Design review of the part built by this model. Coordinates are the model's own, in mm. Face numbers are marked on the shaded views. Round coordinates to 2 decimals unless told otherwise and drop trailing zeros. Loops run counter-clockwise (first coordinate to the right, second up) from the corner with the lowest first, then second, coordinate; pieces in that order, holes last. Notation, with made-up numbers: (46.5, -15) - (84.5, -15) arc R16 ccw to (84.5, 11) - close; hole circle Ø6 at (82.5, 85.5). An arc over 180 degrees is marked (long way). Return JSON: item names as keys, results as strings. Group by question number.
Autodesk Inventor part; units mm, degrees
ref_plane "YZ Plane" through (0, 0, 0) normal (1, 0, 0) x (0, 1, 0)
ref_plane "XZ Plane" through (0, 0, 0) normal (0, 1, 0) x (-1, 0, 0)
ref_plane "XY Plane" through (0, 0, 0) normal (0, 0, 1) x (1, 0, 0)
sketch "スケッチ1" plane through (0, 0, 0) normal (0, 0, 1) x (1, 0, 0)
  circle A0 centre (0, 0) radius 1.5
  dimension "d0" = 3
extrude "押し出し1" add sketch "スケッチ1" along normal blind 12
thread "ねじ1"
sketch "スケッチ2" plane through (0, 0, 12) normal (0, 0, 1) x (1, 0, 0)
  circle A0 centre (0, 0) radius 3
  dimension "d5" = 6
extrude "押し出し2" add sketch "スケッチ2" against normal blind 1.75
chamfer "面取り1" distance 1.5 angle 45 1 edges at (-3, 0, 10.25)
sketch "スケッチ3" plane through (0, 0, 12) normal (0, 0, 1) x (1, 0, 0)
  line L0 (0, 1.1547) -> (1, 0.5774)
  line L1 (1, 0.5774) -> (1, -0.5774)
  line L2 (1, -0.5774) -> (0, -1.1547)
  line L3 (0, -1.1547) -> (-1, -0.5774)
  line L4 (-1, -0.5774) -> (-1, 0.5774)
  line L5 (-1, 0.5774) -> (0, 1.1547)
  point P0 (0, 0)
  point P1 (0, 0)
  dimension "d11" = 2
extrude "押し出し3" cut sketch "スケッチ3" against normal blind 1.5
properties part number "m3皿ネジ12" material "鉄 灰色"
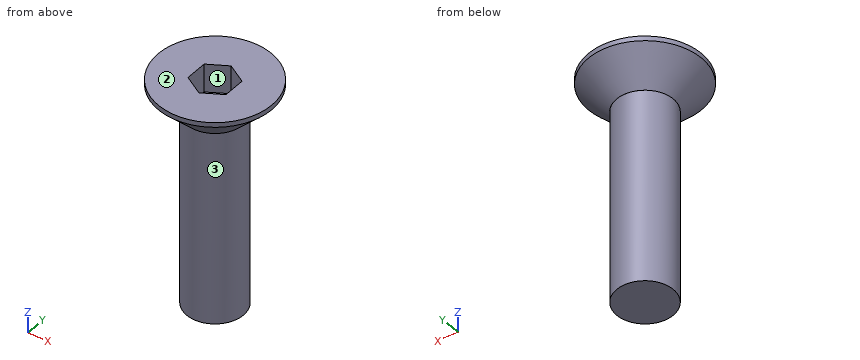
Q1. Draft analysis for pull direction Y (two halves, no side actions). For the marked faces 1, 2 and 3, state which applies: pulls with the +Y half, pulls with the -Y half, needs draft (parallel to the pull), parting line crosses it, or undercut.
Q2. Insertion check: pin 1 Ø3 at (y, z) = (-2, 8) entering from -X; pin 2 Ø0.6 at (y, z) = (0, 11) entering from -X; pin 3 Ø1 at (x, z) = (1, 10.5) entering from +Y. Each pin has a flat end and moves straight along its axis. Give the tip position at first contact, or say it passes through.
Q3. For line 1 (X direction, y = -0.5, z = 0.5); line 2 (Y direction, x = -1.1, z = 11.25); line 3 (Z direction, x = 2.05, y = 0.25), list the stretches that pass through material, from the lowest coordinate up.
Q4. Add section B-B, the plane z = 2. State the section outline as (x, y) points.
Evaluation:
{
 "1": {"face 1": "undercut", "face 2": "needs draft", "face 3": "parting line crosses it"},
 "2": {"pin 1": "x = -1.41", "pin 2": "x = -2.55", "pin 3": "y = 2.06"},
 "3": {"line 1": "-1.41 to 1.41", "line 2": "-2.25 to 2.25", "line 3": "10.81 to 12"},
 "4": {"outline": "circle Ø3 at (0, 0)"}
}
